from build123d import *

# Parameters (mm, degrees)
SKETCH1_R             = 8.334375
BOSS_EXTRUDE1_DEPTH   = 3.0734
F_6_CLEARANCE_HOLE1_D = 3.96875
SKETCH4_R             = 10.715625
SKETCH4_R_2           = 8.334375
BOSS_EXTRUDE2_DEPTH   = 20.6375
CUT_EXTRUDE1_DEPTH    = 26.003125
SKETCH7_W             = 3.96875
SKETCH7_H             = 9.128125
BOSS_EXTRUDE3_DEPTH   = 11.90625
CUT_EXTRUDE2_DEPTH    = 42.671875
F_2_CLEARANCE_HOLE1_D = 2.7051
BOSS_EXTRUDE7_DEPTH   = 0.79375
BOSS_EXTRUDE8_DEPTH   = 0.79375


with BuildPart() as part:
    # Sketch1 → Boss-Extrude1 (new body)
    with BuildSketch(Plane.XY):
        with BuildLine():
            Line((-31.397200262, 6.427931006), (-4.092200262, 23.811056006))
            ThreePointArc((-4.092200262, 23.811056006), (0, 25.003125), (4.092200262, 23.811056006))
            Line((4.092200262, 23.811056006), (31.397200262, 6.427931006))
            ThreePointArc((31.397200262, 6.427931006), (34.925, 0), (31.397200262, -6.427931006))
            Line((31.397200262, -6.427931006), (4.092200262, -23.811056006))
            ThreePointArc((4.092200262, -23.811056006), (0, -25.003125), (-4.092200262, -23.811056006))
            Line((-4.092200262, -23.811056006), (-31.397200262, -6.427931006))
            ThreePointArc((-31.397200262, -6.427931006), (-34.925, 0), (-31.397200262, 6.427931006))
        make_face()
        Circle(SKETCH1_R, mode=Mode.SUBTRACT)
    extrude(amount=BOSS_EXTRUDE1_DEPTH)

    # #6 Clearance Hole1 (through all)
    with Locations(Plane.XY.offset(3.0734)):
        with Locations((-29, 0), (29, 0)):
            Hole(F_6_CLEARANCE_HOLE1_D / 2)

    # Sketch4 → Boss-Extrude2 (add)
    with BuildSketch(Plane.XY.offset(3.0734)):
        Circle(SKETCH4_R)
        Circle(SKETCH4_R_2, mode=Mode.SUBTRACT)
    extrude(amount=BOSS_EXTRUDE2_DEPTH)

    # Sketch6 → Cut-Extrude1 (cut, through all)
    with BuildSketch(Plane(origin=(0, 0, 0), x_dir=(1, 0, 0), z_dir=(0, 1, 0))):
        Polygon((-10.715625, -12.995275), (10.715625, -12.995275), (10.715625, -14.582775), (2.778125, -14.582775), (2.778125, -23.7109), (-2.778125, -23.7109), (-2.778125, -14.582775), (-10.715625, -14.582775), align=None)
    extrude(amount=-CUT_EXTRUDE1_DEPTH, mode=Mode.SUBTRACT)

    # Sketch7 → Boss-Extrude3 (add)
    with BuildSketch(Plane(origin=(0, -7.857724106, 0), x_dir=(1, 0, 0), z_dir=(0, 1, 0))):
        with Locations((-4.7625, -19.1468375)):
            Rectangle(SKETCH7_W, SKETCH7_H)
        with Locations((4.7625, -19.1468375)):
            Rectangle(SKETCH7_W, SKETCH7_H)
    extrude(amount=-BOSS_EXTRUDE3_DEPTH)

    # Sketch8 → Cut-Extrude2 (cut, through all)
    with BuildSketch(Plane.ZY.offset(6.746875)):
        with BuildLine():
            Line((23.7109, -15.199911606), (23.7109, -21.050205541))
            Line((23.7109, -21.050205541), (14.582775, -21.050205541))
            Line((14.582775, -21.050205541), (14.582775, -15.199911606))
            ThreePointArc((14.582775, -15.199911606), (19.1468375, -19.763974106), (23.7109, -15.199911606))
        make_face()
    extrude(amount=-CUT_EXTRUDE2_DEPTH, mode=Mode.SUBTRACT)

    # #2 Clearance Hole1 (through all)
    with Locations(Plane.ZY.offset(6.746875)):
        with Locations((19.1468375, -15.199911606)):
            Hole(F_2_CLEARANCE_HOLE1_D / 2)

    # Sketch11 → Boss-Extrude7 (add, symmetric)
    with BuildSketch(Plane(origin=(0, 0, 0), x_dir=(1, 0, 0), z_dir=(0, 1, 0))):
        Polygon((-10.461625, -12.995275), (-12.842875, -12.995275), (-23.161625, -3.0734), (-10.461625, -3.0734), align=None)
        Polygon((23.161625, -3.0734), (10.461625, -3.0734), (10.461625, -12.995275), (12.842875, -12.995275), align=None)
    extrude(amount=BOSS_EXTRUDE7_DEPTH, both=True)

    # Sketch13 → Boss-Extrude8 (add, symmetric)
    with BuildSketch(Plane(origin=(0, 0, 0), x_dir=(0, 0, -1), z_dir=(1, 0, 0))):
        Polygon((-12.995275, 10.377516644), (-12.995275, 12.758766644), (-3.0734, 23.077516644), (-3.0734, 10.377516644), align=None)
        Polygon((-3.0734, -23.077516644), (-3.0734, -10.377516644), (-12.995275, -10.377516644), (-12.995275, -12.758766644), align=None)
    extrude(amount=BOSS_EXTRUDE8_DEPTH, both=True)


solid = part.part
Model file for the job. Use its own axes, mm. A direction names the side the tool comes from. Give positions to 0.01 mm unless a question says otherwise; leave off trailing zeros. Loops run counter-clockwise (first coordinate to the right, second up) from the corner with the lowest first, then second, coordinate; pieces in that order, holes last.
Item 1: Drop flat-ended pins along their axis: P1, Ø4.5, axis at y = -15.5, z = 19, coming from the +X side; P2, Ø0.5, axis at x = 0, y = 11.5, coming from the +Z side; P3, Ø1.7, axis at x = -9, z = 13.5, coming from the -Y side; P4, Ø21.5, axis at x = 0, y = 0, coming from the +Z side. Give the stop position or say it passes through.
Check values:
P1: stops at x = 6.75
P2: stops at z = 13
P3: stops at y = -6.76
P4: stops at z = 23.71
Item 2: Which spindle directions (+Z, -Z, +X, -X, +Y, -Y) get a long thin tool onto all of the face, cutting with end or side? Do faces 1 (the face through (15, -0.794, 7)), 2 (the face through (-2.778, -12, 19)), 3 (the face through (0.794, 16, 7)), 4 (the face through (10, 0, 14)). Say none if no direction does.
Check values:
face 1: +Z, +X, -Y
face 2: +Z, -Y
face 3: +Z, +X, +Y
face 4: +X, -X, -Y
Item 3: Slice it at D-D (y = 9.5). Write the cut outline in (x, z), plus the area to 3 significant figures.
Check values:
outline: (-26.57, 0) - (26.57, 0) - (26.57, 3.07) - (4.96, 3.07) - (4.96, 23.71) - (-4.96, 23.71) - (-4.96, 3.07) - (-26.57, 3.07) - close
area: 368 mm2
Item 4: Drill centre lines: line 1 along X through (y, z) = (0, 18.75); line 2 along X through (y, z) = (-15.5, 15.75); line 3 along Z through (x, y) = (-6, -7). Where is each one in solid material? Low to high.
Check values:
line 1: x = -10.72 to -8.33, 8.33 to 10.72
line 2: x = -6.75 to -2.78, 2.78 to 6.75
line 3: z = 0 to 13, 14.58 to 23.71
Item 5: Slice it at A-A (x = -7.5). Write the cut outline in (y, z).
Check values:
outline: (-21.64, 0) - (-3.63, 0) - (-3.63, 13) - (-7.65, 13) - (-7.65, 3.07) - (-21.64, 3.07) - close; (-7.65, 14.58) - (-3.63, 14.58) - (-3.63, 23.71) - (-7.65, 23.71) - close; (3.63, 0) - (21.64, 0) - (21.64, 3.07) - (7.65, 3.07) - (7.65, 23.71) - (3.63, 23.71) - close
Item 6: Slice it at B-B (x = 29). Write the cut outline in (y, z).
Check values:
outline: (-7.95, 0) - (-1.98, 0) - (-1.98, 3.07) - (-7.95, 3.07) - close; (1.98, 0) - (7.95, 0) - (7.95, 3.07) - (1.98, 3.07) - close
Item 7: Mould opens along Y. For faces 5 (the face through (15, 0.794, 7)), 6 (the face through (-6.747, -13, 19)), 7 (the face through (34.924, 0.107, 1.515)), 8 (the face through (-4.73, -13.86, 19.32)) say: +Y half, -Y half, draft (parallel to the pull), parting line (faces both ways), or undercut.
Check values:
face 5: +Y half
face 6: draft
face 7: parting line
face 8: undercut
Item 8: Slice it at C-C (z = 19.5). Write the cut outline in (x, y), plus the area to 3 significant figures.
Check values:
outline: (-6.75, -19.75) - (-2.78, -19.75) - (-2.78, -16.51) - (-6.75, -16.51) - close; (-6.75, -13.89) - (-2.78, -13.89) - (-2.78, -7.86) arc R8.33 cw (long way) to (2.78, -7.86) - (2.78, -13.89) - (6.75, -13.89) - (6.75, -8.32) arc R10.72 ccw (long way) to (-6.75, -8.32) - close; (2.78, -19.75) - (6.75, -19.75) - (6.75, -16.51) - (2.78, -16.51) - close
area: 190 mm2
